Geometry: final body of the model. Coordinates: model frame, mm. A direction names the side the tool comes from. Round coordinates to 2 decimals unless told otherwise and drop trailing zeros. Write each loop counter-clockwise with the first axis right and the second up, starting at its lowest first coordinate (ties: lowest second). Pieces come first, ordered by that corner, then holes. Notation, with made-up numbers: M -28,33 L -23,33 A27 ccw -23,49 Z; hole C 55.5,58.25 d11. An arc over 180 degrees is marked long. Use one line per item in the form item = value. Start each with the question number.
from build123d import *

# Parameters (mm, degrees)
BOSS_EXTRUDE1_DEPTH  = 6.35
FILLET1_R            = 8.5
FILLET2_R            = 10
M5_CLEARANCE_HOLE1_D = 5.5
M3_CLEARANCE_HOLE1_D = 3.4
CUT_EXTRUDE1_DEPTH   = 7.35
SKETCH9_W            = 3
SKETCH9_H            = 12
BOSS_EXTRUDE2_DEPTH  = 6.35
CUT_EXTRUDE2_DEPTH   = 7.35
FILLET3_R            = 1
FILLET4_R            = 3


with BuildPart() as part:
    # Sketch1 → Boss-Extrude1 (new body)
    with BuildSketch(Plane(origin=(0, 0, 0), x_dir=(1, 0, 0), z_dir=(0, 1, 0))):
        Polygon((38.1, -25.4), (-38.1, -25.4), (-38.1, -45.04), (-59.74, -45.04), (-59.74, 25.4), (-38.1, 25.4), (38.1, 25.4), align=None)
    extrude(amount=BOSS_EXTRUDE1_DEPTH)

    # Fillet1
    fillet1_edges = [part.edges().sort_by_distance(p)[0] for p in [
        (-38.1, 3.175, 45.04),
        (-59.74, 3.175, 45.04),
    ]]
    fillet(fillet1_edges, radius=FILLET1_R)

    # Fillet2
    fillet2_edges = [part.edges().sort_by_distance(p)[0] for p in [
        (38.1, 3.175, -25.4),
        (38.1, 3.175, 25.4),
        (-59.74, 3.175, -25.4),
    ]]
    fillet(fillet2_edges, radius=FILLET2_R)

    # M5 Clearance Hole1 (through all)
    with Locations(Plane(origin=(0, 6.35, 0), x_dir=(-1, 0, 0), z_dir=(0, 1, 0))):
        with Locations((0, 12.7), (-25.4, 12.7), (-25.4, -12.7), (0, -12.7)):
            Hole(M5_CLEARANCE_HOLE1_D / 2)

    # M3 Clearance Hole1 (through all)
    with Locations(Plane(origin=(0, 6.35, 0), x_dir=(-1, 0, 0), z_dir=(0, 1, 0))):
        with Locations((15.4, 10), (15.4, -10), (35.4, -10), (35.4, 10)):
            Hole(M3_CLEARANCE_HOLE1_D / 2)

    # Sketch8 → Cut-Extrude1 (cut, through all)
    with BuildSketch(Plane(origin=(0, 6.35, 0), x_dir=(1, 0, 0), z_dir=(0, 1, 0))):
        with BuildLine():
            Line((-51.61383297, -8.23383297), (-49.97383297, -9.87383297))
            ThreePointArc((-49.97383297, -9.87383297), (-46.22616703, -9.87383297), (-46.22616703, -6.12616703))
            Line((-46.22616703, -6.12616703), (-47.86616703, -4.48616703))
            ThreePointArc((-47.86616703, -4.48616703), (-51.61383297, -4.48616703), (-51.61383297, -8.23383297))
        make_face()
        with BuildLine():
            Line((-47.86616703, -36.91383297), (-46.22616703, -35.27383297))
            ThreePointArc((-46.22616703, -35.27383297), (-46.22616703, -31.52616703), (-49.97383297, -31.52616703))
            Line((-49.97383297, -31.52616703), (-51.61383297, -33.16616703))
            ThreePointArc((-51.61383297, -33.16616703), (-51.61383297, -36.91383297), (-47.86616703, -36.91383297))
        make_face()
    extrude(amount=-CUT_EXTRUDE1_DEPTH, mode=Mode.SUBTRACT)

    # Sketch9 → Boss-Extrude2 (add)
    with BuildSketch(Plane(origin=(0, 6.35, 0), x_dir=(1, 0, 0), z_dir=(0, 1, 0))):
        with Locations((-14.05, 31.4)):
            Rectangle(SKETCH9_W, SKETCH9_H)
        with Locations((-36.75, 31.4)):
            Rectangle(SKETCH9_W, SKETCH9_H)
        with Locations((-36.75, -31.4)):
            Rectangle(SKETCH9_W, SKETCH9_H)
        with Locations((-14.05, -31.4)):
            Rectangle(SKETCH9_W, SKETCH9_H)
    extrude(amount=-BOSS_EXTRUDE2_DEPTH)

    # Sketch10 → Cut-Extrude2 (cut, through all)
    with BuildSketch(Plane(origin=(0, 6.35, 0), x_dir=(1, 0, 0), z_dir=(0, 1, 0))):
        Polygon((-33.75, 12.4), (-30.55, 12.4), (-30.55, 19.8), (-29.3, 19.8), (-29.3, 22.4), (-30.55, 22.4), (-30.55, 25.4), (-33.75, 25.4), (-33.75, 22.4), (-35, 22.4), (-35, 19.8), (-33.75, 19.8), align=None)
        Polygon((-20.25, 12.4), (-20.25, 19.8), (-21.5, 19.8), (-21.5, 22.4), (-20.25, 22.4), (-20.25, 25.4), (-17.05, 25.4), (-17.05, 22.4), (-15.8, 22.4), (-15.8, 19.8), (-17.05, 19.8), (-17.05, 12.4), align=None)
        Polygon((-20.25, -22.4), (-20.25, -25.4), (-17.05, -25.4), (-17.05, -22.4), (-15.8, -22.4), (-15.8, -19.8), (-17.05, -19.8), (-17.05, -12.4), (-20.25, -12.4), (-20.25, -19.8), (-21.5, -19.8), (-21.5, -22.4), align=None)
        Polygon((-30.55, -22.4), (-30.55, -25.4), (-33.75, -25.4), (-33.75, -22.4), (-35, -22.4), (-35, -19.8), (-33.75, -19.8), (-33.75, -12.4), (-30.55, -12.4), (-30.55, -19.8), (-29.3, -19.8), (-29.3, -22.4), align=None)
    extrude(amount=-CUT_EXTRUDE2_DEPTH, mode=Mode.SUBTRACT)

    # Fillet3
    fillet3_edges = [part.edges().sort_by_distance(p)[0] for p in [
        (-15.55, 3.175, -37.4),
        (-12.55, 3.175, -37.4),
        (-38.25, 3.175, -37.4),
        (-35.25, 3.175, -37.4),
        (-38.143617795, 3.175, 37.4),
        (-35.25, 3.175, 37.4),
        (-12.55, 3.175, 37.4),
        (-15.55, 3.175, 37.4),
        (-30.55, 3.175, -19.8),
        (-33.75, 3.175, -19.8),
        (-33.75, 3.175, -25.4),
        (-30.55, 3.175, -25.4),
        (-20.25, 3.175, -19.8),
        (-20.25, 3.175, -25.4),
        (-17.05, 3.175, -25.4),
        (-17.05, 3.175, -19.8),
        (-20.25, 3.175, 19.8),
        (-17.05, 3.175, 19.8),
        (-17.05, 3.175, 25.4),
        (-20.25, 3.175, 25.4),
        (-30.55, 3.175, 25.4),
        (-33.75, 3.175, 25.4),
        (-33.75, 3.175, 19.8),
        (-30.55, 3.175, 19.8),
    ]]
    fillet(fillet3_edges, radius=FILLET3_R)

    # Fillet4
    fillet4_edges = [part.edges().sort_by_distance(p)[0] for p in [
        (-12.55, 3.175, -25.4),
        (-38.25, 3.175, -25.4),
        (-12.55, 3.175, 25.4),
    ]]
    fillet(fillet4_edges, radius=FILLET4_R)


solid = part.part
1. Set-up query: faces 4 (the face through (-33.75, 3, -23)), 5 (the face through (10, 3, -25.4)), 6 (the face through (-30.55, 3, 16)), 7 (the face through (-29.3, 3, -21)). Return all of +Z, -Z, +X, -X, +Y, -Y with unobstructed straight access to the full face (end or side cutting, diameter ignored); none if empty.
2. Section query D-D (x = -0.5). Return loops of the section in (y, z).
3. Pull-direction query (X, two-part tool) for faces 1 (the face through (-59.74, 3, 11)), 2 (the face through (-0.358, 3.131, 15.427)), 3 (the face through (-11.65, 3.13, 26.26)); classes: released by +X, released by -X, zero draft, split by the parting line, or undercut.
4. Contact query for flat-ended pins moving along their axis: pin 1 (0.6 mm diameter, centred on x = -16, y = 4.5, fed in from +Z); pin 2 (0.6 mm diameter, centred on y = 4.5, z = -23.5, fed in from -X); pin 3 (3 mm diameter, centred on y = 4, z = 31, fed in from +X); pin 4 (6.5 mm diameter, centred on x = 0, z = 12.7, fed in from -Y). Output: stop coordinate, or through.
5. Section query B-B (z = 14). Return loops of the section in (x, y), then the cut area to 3 significant figures.
6. Section query C-C (y = 3). Give the number of separate pieces and of enclosed holes in the cut face, then the cut area to 3 significant figures.
7. Section query A-A (x = 25.4). Return loops of the section in (y, z).
8. Ray query, probe 1 along Z at (x, y) = (0, 4.25); probe 2 along X at (y, z) = (6, 16); probe 3 along Z at (x, y) = (-15.4, 1.75). Return the intervals inside material, ascending.
Checks:
q1.face_4 = -Z, +Y, -Y
q1.face_5 = -Z, +X, +Y, -Y
q1.face_6 = +Z, +Y, -Y
q1.face_7 = +Y, -Y
q2.outline = M 0,-25.4 L 6.35,-25.4 L 6.35,-15.4 L 0,-15.4 Z; M 0,-10 L 6.35,-10 L 6.35,10 L 0,10 Z; M 0,15.4 L 6.35,15.4 L 6.35,25.4 L 0,25.4 Z
q3.face_1 = released by -X
q3.face_2 = undercut
q3.face_3 = released by +X
q4.pin_1 = 25.4
q4.pin_2 = -56
q4.pin_3 = -12.55
q4.pin_4 = 0
q5.outline = M -59.74,0 L -33.75,0 L -33.75,6.35 L -59.74,6.35 Z; M -30.55,0 L -20.25,0 L -20.25,6.35 L -30.55,6.35 Z; M -17.05,0 L -2.42,0 L -2.42,6.35 L -17.05,6.35 Z; M 2.42,0 L 22.98,0 L 22.98,6.35 L 2.42,6.35 Z; M 27.82,0 L 38.1,0 L 38.1,6.35 L 27.82,6.35 Z
q5.area = 519 mm^2
q6.separate_pieces = 1
q6.enclosed_holes = 10
q6.area = 5,050 mm^2
q7.outline = M 0,-25.4 L 6.35,-25.4 L 6.35,-15.45 L 0,-15.45 Z; M 0,-9.95 L 6.35,-9.95 L 6.35,9.95 L 0,9.95 Z; M 0,15.45 L 6.35,15.45 L 6.35,25.4 L 0,25.4 Z
q8.probe_1 = -25.4 to -15.45, -9.95 to 9.95, 15.45 to 25.4
q8.probe_2 = -59.74 to -33.75, -30.55 to -20.25, -17.05 to 38.08
q8.probe_3 = -36.93 to -11.7, -8.3 to 8.3, 11.7 to 36.93
